The model under review builds one solid part; all positions refer to its coordinate system, in mm. Face numbers are marked on the shaded views. A direction names the side the tool comes from. Give positions to 0.01 mm unless a question says otherwise; leave off trailing zeros. Order: outer loops, then holes, each group sorted by start corner. A loop starts at its lowest first (then second) coordinate and runs counter-clockwise, first axis right, second up.
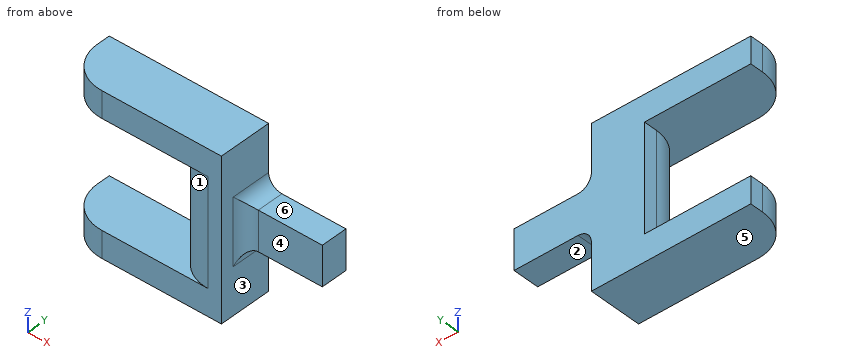
```python
from build123d import *

# Parameters (mm, degrees)
F1_DEPTH = 20
F2_R     = 15
F3_W     = 30.964084
F3_H     = 14.88658
F4_DEPTH = 10
F5_R     = 5


with BuildPart() as f1:
    # F0 (on Front) → F1 (new body)
    with BuildSketch(Plane.XZ):
        Polygon((30, 30), (-30, 30), (-30, 20.051985), (10, 20.051985), (10, -19.948015), (-30, -19.948015), (-30, -30), (30, -30), align=None)
    extrude(amount=F1_DEPTH)

    # F2
    f2_edges = [f1.edges().sort_by_distance(p)[0] for p in [
        (10, -20, 0.051985),
        (-30, -20, -24.974007),
        (-30, -20, 25.025993),
    ]]
    fillet(f2_edges, radius=F2_R)

    # F3 (on Front) → F4 (join)
    with BuildSketch(Plane.XZ):
        with Locations((43.617677, 0)):
            Rectangle(F3_W, F3_H)
    extrude(amount=F4_DEPTH)

    # F5
    f5_edges = [f1.edges().sort_by_distance(p)[0] for p in [
        (30, -5, 7.44329),
        (30, -10, 0),
        (30, -5, -7.44329),
    ]]
    fillet(f5_edges, radius=F5_R)


solid = f1.part
```
Item 1: For line 1 (Z direction, x = 5, y = -12.75); line 2 (Y direction, x = 43, z = 0); line 3 (X direction, y = -5.5, z = -2.5), list the stretches that pass through material, from the lowest coordinate up.
Values found:
line 1: z = -30 to -19.95, 20.05 to 30
line 2: y = -10 to 0
line 3: x = 10.01 to 59.1
Item 2: For the marked faces 4, 5 and 6, list the 3-axis set-ups (+Z, -Z, +X, -X, +Y, -Y) from which the entire face can be reached by the end or side of a thin tool; tool diameter is ignored.
Values found:
face 4: +Z, -Z, +X, -Y
face 5: -Z, +X, -X, +Y, -Y
face 6: +Z, +X, +Y, -Y
Item 3: Take a section at B-B (z = 2). Give the boundary of the cut face in (x, y), and give its area (3 significant figures).
Values found:
outline: (10, -5) arc R15 ccw to (25, -20) - (30, -20) - (30, -15) arc R5 cw to (35, -10) - (59.1, -10) - (59.1, 0) - (10, 0) - close
area: 648 mm2
Item 4: Draft analysis for pull direction Z (two halves, no side actions). For the marked faces 1, 2 and 3, state which applies: released by +Z, released by -Z, zero draft, split by the parting line, or undercut.
Values found:
face 1: undercut
face 2: released by -Z
face 3: zero draft
Item 5: Take a section at C-C (y = -3). Give the boundary of the cut face in (x, z).
Values found:
outline: (-30, -30) - (30, -30) - (30, -12.44) arc R5 cw to (35, -7.44) - (59.1, -7.44) - (59.1, 7.44) - (35, 7.44) arc R5 cw to (30, 12.44) - (30, 30) - (-30, 30) - (-30, 20.05) - (10, 20.05) - (10, -19.95) - (-30, -19.95) - close
Item 6: Clearance check with flat-ended pins moving along their axes: pin 1 Ø12 at (y, z) = (-13.5, 6) entering from -X; pin 2 Ø2 at (y, z) = (-6.5, 22.5) entering from -X; pin 3 Ø8 at (x, y) = (51.5, -6.5) entering from -Z. State where each tip first meets the part, or that it passes through.
Values found:
pin 1: stops at x = 10.21
pin 2: stops at x = -29.99
pin 3: stops at z = -7.44
Item 7: Take a section at D-D (x = 20.5). Give the boundary of the cut face in (y, z).
Values found:
outline: (-20, -30) - (0, -30) - (0, 30) - (-20, 30) - (-20, 20.05) - (-19.31, 20.05) - (-19.31, -19.95) - (-20, -19.95) - close
Item 8: Take a section at A-A (x = -5). Give the boundary of the cut face in (y, z), and give its area (3 significant figures).
Values found:
outline: (-20, -30) - (0, -30) - (0, -19.95) - (-20, -19.95) - close; (-20, 20.05) - (0, 20.05) - (0, 30) - (-20, 30) - close
area: 400 mm2
